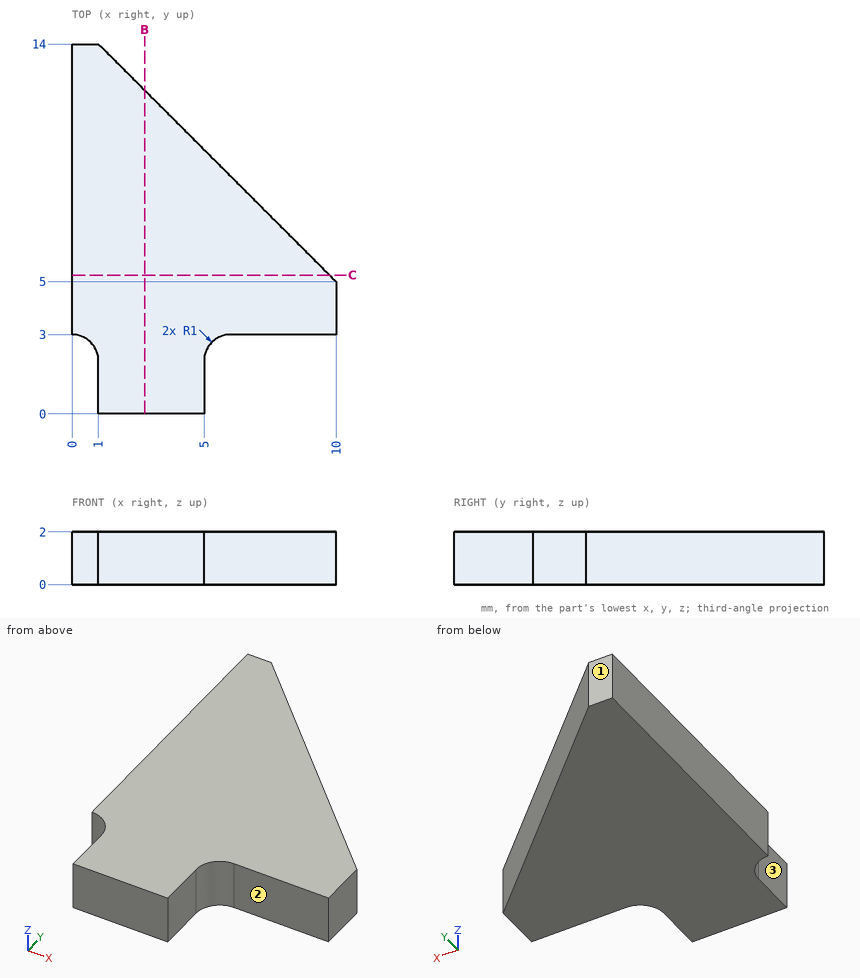
Source: three-view drawing plus pictorial views. Frame: mm from the lowest corner of the part. A direction names the side the tool comes from. Give positions to 0.01 mm unless a question says otherwise; leave off trailing zeros. Loops run counter-clockwise (first coordinate to the right, second up) from the corner with the lowest first, then second, coordinate; pieces in that order, holes last.
1) Section query C-C on y = 5.25. Return the cut outline in (x, z).
A:
outline: (0, 0) - (9.75, 0) - (9.75, 2) - (0, 2) - close
2) Reachability of the marked faces 1, 2 and 3 from +Z, -Z, +X, -X, +Y, -Y: full face, straight path, thin tool, end or side. Return the list, or none.
A:
face 1: +Z, -Z, +X, -X, +Y
face 2: +Z, -Z, +X, -Y
face 3: +Z, -Z, -X, -Y
3) Section query B-B on x = 2.75. Return the cut outline in (y, z).
A:
outline: (0, 0) - (12.25, 0) - (12.25, 2) - (0, 2) - close
4) Contact query for flat-ended pins moving along their axis: pin 1 (1 mm diameter, centred on x = 9, z = 1.5, fed in from -Y); pin 2 (0.6 mm diameter, centred on y = 1, z = 1, fed in from +X). Output: stop coordinate, or through.
A:
pin 1: stops at y = 3
pin 2: stops at x = 5
5) Line query: L1, parallel to X at y = 1, z = 1.35; L2, parallel to X at y = 9, z = 0.85; L3, parallel to Y at x = 2.25, z = 0.4. Output: solid intervals per line, ascending.
A:
L1: x = 1 to 5
L2: x = 0 to 6
L3: y = 0 to 12.75
